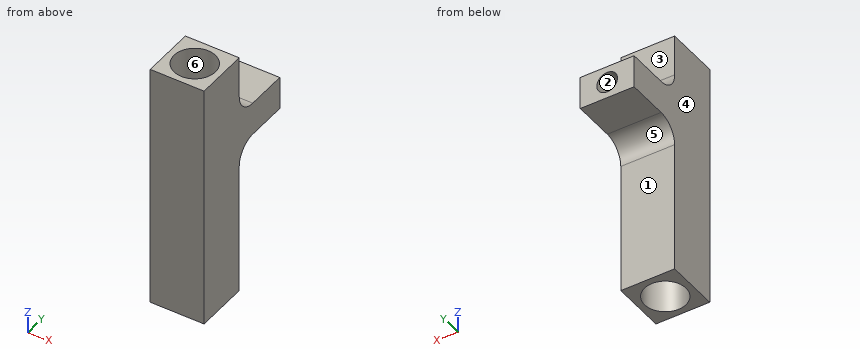
from build123d import *

# Parameters (mm, degrees)
BOSS_EXTRUDE1_DEPTH            = 13
BOSS_EXTRUDE1_DEPTH_BACK       = 13
CUT_EXTRUDE1_REACH             = 111.627
SKETCH1_R                      = 10
CUT_EXTRUDE1_DIRECTION_2_REACH = 111.627
CUT_EXTRUDE2_REACH             = 117.347
CUT_EXTRUDE2_END_RADIUS        = 10
SKETCH3_R                      = 5


with BuildPart() as part:
    # Sketch2 → Boss-Extrude1 (new, two sides: drawn at the far end of the back side and taken through both)
    with BuildSketch(Plane(origin=(0, 0, 0), x_dir=(0, 0, -1), z_dir=(1, 0, 0)).offset(-BOSS_EXTRUDE1_DEPTH_BACK)):
        with BuildLine():
            Line((36, 13), (100, 13))
            Line((100, 13), (100, -13))
            Line((100, -13), (0, -13))
            Line((0, -13), (-20, -13))
            Line((-20, -13), (-20, 13))
            Line((-20, 13), (0, 13))
            ThreePointArc((0, 13), (7.071067812, 15.928932188), (10, 23))
            Line((10, 23), (10, 43))
            Line((10, 43), (26, 43))
            Line((26, 43), (26, 23))
            ThreePointArc((26, 23), (28.928932188, 15.928932188), (36, 13))
        make_face()
    extrude(amount=BOSS_EXTRUDE1_DEPTH + BOSS_EXTRUDE1_DEPTH_BACK)

    # Cut-Extrude1: up to this face of the body (flat: up to its plane)
    cut_extrude1_end = Plane(part.part.faces().sort_by_distance((0, 0, -100))[0])
    # Sketch1 → Cut-Extrude1 (cut, up to the picked face)
    with BuildSketch(Plane.XY, mode=Mode.PRIVATE) as cut_extrude1_sk1:
        Circle(SKETCH1_R)
    cut_extrude1_tool1 = split(extrude(cut_extrude1_sk1.sketch, amount=-CUT_EXTRUDE1_REACH, mode=Mode.PRIVATE), bisect_by=cut_extrude1_end, keep=Keep.BOTH, mode=Mode.PRIVATE)
    add(cut_extrude1_tool1.solids().sort_by(Axis((0, 0, 0), (0, 0, -1)))[0], mode=Mode.SUBTRACT)

    # Cut-Extrude1 direction 2: up to this face of the body (flat: up to its plane)
    cut_extrude1_direction_2_end = Plane(part.part.faces().sort_by_distance((0, 0, 20))[0])
    # Sketch1 → Cut-Extrude1 direction 2 (cut, up to the picked face)
    with BuildSketch(Plane.XY, mode=Mode.PRIVATE) as cut_extrude1_direction_2_sk1:
        Circle(SKETCH1_R)
    cut_extrude1_direction_2_tool1 = split(extrude(cut_extrude1_direction_2_sk1.sketch, amount=CUT_EXTRUDE1_DIRECTION_2_REACH, mode=Mode.PRIVATE), bisect_by=cut_extrude1_direction_2_end, keep=Keep.BOTH, mode=Mode.PRIVATE)
    add(cut_extrude1_direction_2_tool1.solids().sort_by(Axis((0, 0, 0), (0, 0, 1)))[0], mode=Mode.SUBTRACT)

    # Cut-Extrude2: up to this cylinder (the profile starts outside it)
    cut_extrude2_end = Plane(origin=(0, 0, -18), z_dir=(0, 0, 1)) * Cylinder(CUT_EXTRUDE2_END_RADIUS, 255.694, mode=Mode.PRIVATE)
    # Sketch3 → Cut-Extrude2 (cut, up to the surface)
    with BuildSketch(Plane(origin=(0, 43, 0), x_dir=(1, 0, 0), z_dir=(0, 1, 0)), mode=Mode.PRIVATE) as cut_extrude2_sk1:
        with Locations(Location((0, 18, 0), (0, 0, 270))):
            Circle(SKETCH3_R)
    cut_extrude2_tool1 = extrude(cut_extrude2_sk1.sketch, amount=-CUT_EXTRUDE2_REACH, mode=Mode.PRIVATE) - cut_extrude2_end
    add(cut_extrude2_tool1.solids().sort_by_distance((0, 43, -18))[0], mode=Mode.SUBTRACT)


solid = part.part
Read the model definition and answer for the solid it produces. Units are mm, in the model's axes. Face numbers are marked on the shaded views. A direction names the side the tool comes from. Give positions to 0.01 mm unless a question says otherwise; leave off trailing zeros. Loops run counter-clockwise (first coordinate to the right, second up) from the corner with the lowest first, then second, coordinate; pieces in that order, holes last. Notation, with made-up numbers: M 1,12.25 L 54,12.25 A24 ccw 54,47.25 Z; hole C -6.5,27.25 d10. An arc over 180 degrees is marked long. Write each question's results on one line, items separated by ' | '.
1. A tool of negligible diameter and unlimited length cuts with its end or side. For the marked faces 1, 2 and 3, from which of +Z, -Z, +X, -X, +Y, -Y can it reach the whole face along a straight path? Write none if from no direction.
Values:
face 1: -Z, +X, -X, +Y | face 2: +Y | face 3: +Z, +X, -X, +Y
2. Section C-C on x = -8 is taken. Give the vertices of the cut face in (y, z).
Values:
outline: M -13,-100 L -6,-100 L -6,20 L -13,20 Z; M 6,-100 L 13,-100 L 13,-36 A10 cw 23,-26 L 43,-26 L 43,-10 L 23,-10 A10 cw 13,0 L 13,20 L 6,20 Z
3. The mould has two halves that part along X. Classify the marked faces 4, 5 and 6: pulls with the +X half, pulls with the -X half, needs draft (parallel to the pull), parting line crosses it, or undercut.
Values:
face 4: pulls with the -X half | face 5: needs draft | face 6: undercut
4. Given pin 1 (6 mm diameter, centred on x = -4.5, z = 7, fed in from +Y); pin 2 (6 mm diameter, centred on x = 2.5, y = 30, fed in from -Z); pin 3 (6 mm diameter, centred on x = 4.5, y = 33, fed in from +Z), each flat-ended and moving along its own axis, determine where each tip first touches the part or whether it passes through.
Values:
pin 1: stops at y = 13 | pin 2: stops at z = -26 | pin 3: stops at z = -10
5. Section A-A on x = 0 is taken. Give the vertices of the cut face in (y, z).
Values:
outline: M -13,-100 L -10,-100 L -10,20 L -13,20 Z; M 10,-100 L 13,-100 L 13,-36 A10 cw 23,-26 L 43,-26 L 43,-23 L 10,-23 Z; M 10,-13 L 43,-13 L 43,-10 L 23,-10 A10 cw 13,0 L 13,20 L 10,20 Z
6. Section D-D on z = -30 is taken. Give the vertices of the cut face in (x, y), plus the area to 3 significant figures.
Values:
outline: M -13,-13 L 13,-13 L 13,15 L -13,15 Z; hole C 0,0 d20 | area: 414 mm^2
7. Straight lines are drawn through the part: line 1 (Z direction, x = 0, y = 23); line 2 (X direction, y = 0, z = -44); line 3 (X direction, y = 18, z = -18). For each, find the intervals that lie inside material, in ascending order. Write a range as [from, to].
Values:
line 1: z = [-26, -23], [-13, -10] | line 2: x = [-13, -10], [10, 13] | line 3: x = [-13, -5], [5, 13]
8. Section B-B on y = 1.5 is taken. Give the vertices of the cut face in (x, z), plus the area to 3 significant figures.
Values:
outline: M -13,-100 L -9.89,-100 L -9.89,20 L -13,20 Z; M 9.89,-100 L 13,-100 L 13,20 L 9.89,20 Z | area: 747 mm^2
